For this review, take the finished solid that the model builds, in its own axes (mm). Face numbers are marked on the shaded views. A direction names the side the tool comes from. Round coordinates to 2 decimals unless told otherwise and drop trailing zeros. Loops run counter-clockwise (first coordinate to the right, second up) from the corner with the lowest first, then second, coordinate; pieces in that order, holes last.
1. Clearance check with flat-ended pins moving along their axes: pin 1 Ø13 at (x, z) = (35, 65) entering from +Y; pin 2 Ø1 at (x, z) = (-17.5, 28.5) entering from -Y; pin 3 Ø10 at (x, y) = (0, 0) entering from +Z; pin 4 Ø4 at (y, z) = (11, 114) entering from -X. State where each tip first meets the part, or that it passes through.
2. Consider section A-A on x = 0. State the section outline as (y, z) points.
3. Draft analysis for pull direction Y (two halves, no side actions). For the marked faces 4, 5 and 6, state which applies: released by +Y, released by -Y, zero draft, split by the parting line, or undercut.
4. Tool access review of the marked faces 1, 2 and 3: name each direction out of +Z, -Z, +X, -X, +Y, -Y from which nothing blocks a thin tool from reaching the whole face with its end or side.
5. Consider section C-C on y = 0. State the section outline as (x, z) points, then the cut area to 3 significant figures.
6. Consider section B-B on z = 65. State the section outline as (x, y) points.
7. To check wall thickness, follow line 1 along X through (y, z) = (46, 65); line 2 along Y through (x, z) = (-0.5, 136.5); line 3 along Z through (x, y) = (-2.5, 46). State the ranges of each line that lie inside material, in increasing order.
8. Consider section D-D on x = 35. State the section outline as (y, z) points.
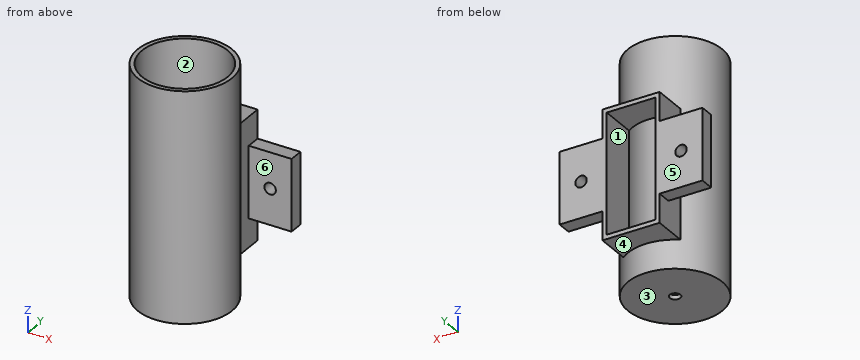
from build123d import *

# Parameters (mm, degrees)
SKETCH_1_R           = 33
EXTRUDE_1_DEPTH      = 160
SHELL_1_T            = -3
EXTRUDE_2_REACH      = 185.243
EXTRUDE_2_END_RADIUS = 33
SKETCH_2_W           = 40
SKETCH_2_H           = 90
SKETCH_3_W           = 34
SKETCH_3_H           = 84
CUT_EXTRUDE_1_DEPTH  = 60
SKETCH_4_W           = 50
SKETCH_4_H           = 10
EXTRUDE_3_DEPTH      = 30
SKETCH_5_R           = 4
CUT_EXTRUDE_2_DEPTH  = 30
SKETCH_6_W           = 50
SKETCH_6_H           = 10
EXTRUDE_4_DEPTH      = 30
SKETCH_7_R           = 4
CUT_EXTRUDE_3_DEPTH  = 30
SKETCH_8_R           = 3.75
CUT_EXTRUDE_4_DEPTH  = 10


with BuildPart() as part:
    # 草图1 → 凸台-拉伸1 (new body)
    with BuildSketch(Plane.XY):
        Circle(SKETCH_1_R)
    extrude(amount=EXTRUDE_1_DEPTH)

    # 抽壳1
    shell_1_openings = [part.faces().sort_by_distance(p)[0] for p in [
        (0, 0, 160),
    ]]
    offset(amount=SHELL_1_T, openings=shell_1_openings, kind=Kind.INTERSECTION)

    # 凸台-拉伸2: up to this cylinder (the profile starts outside it)
    extrude_2_end = Plane(origin=(0, 0, 65), z_dir=(0, 0, -1)) * Cylinder(EXTRUDE_2_END_RADIUS, 437.486, mode=Mode.PRIVATE)
    # 草图2 → 凸台-拉伸2 (add, up to the surface)
    with BuildSketch(Plane(origin=(0, 50, 0), x_dir=(1, 0, 0), z_dir=(0, 1, 0)), mode=Mode.PRIVATE) as extrude_2_sk1:
        with Locations((0, -65)):
            Rectangle(SKETCH_2_W, SKETCH_2_H)
    extrude_2_tool1 = extrude(extrude_2_sk1.sketch, amount=-EXTRUDE_2_REACH, mode=Mode.PRIVATE) - extrude_2_end
    add(extrude_2_tool1.solids().sort_by_distance((0, 50, 65))[0])

    # 草图3 → 切除-拉伸1 (cut)
    with BuildSketch(Plane(origin=(0, 50, 0), x_dir=(1, 0, 0), z_dir=(0, 1, 0))):
        with Locations((0, -65)):
            Rectangle(SKETCH_3_W, SKETCH_3_H)
    extrude(amount=-CUT_EXTRUDE_1_DEPTH, mode=Mode.SUBTRACT)

    # 草图4 → 凸台-拉伸3 (add)
    with BuildSketch(Plane.ZY.offset(20)):
        with Locations((65, 45)):
            Rectangle(SKETCH_4_W, SKETCH_4_H)
    extrude(amount=EXTRUDE_3_DEPTH)

    # 草图5 → 切除-拉伸2 (cut)
    with BuildSketch(Plane(origin=(0, 50, 0), x_dir=(1, 0, 0), z_dir=(0, 1, 0))):
        with Locations(Location((-35, -65, 0), (0, 0, 270))):
            Circle(SKETCH_5_R)
    extrude(amount=-CUT_EXTRUDE_2_DEPTH, mode=Mode.SUBTRACT)

    # 草图6 → 凸台-拉伸4 (add)
    with BuildSketch(Plane(origin=(20, 0, 0), x_dir=(0, 0, -1), z_dir=(1, 0, 0))):
        with Locations((-65, 45)):
            Rectangle(SKETCH_6_W, SKETCH_6_H)
    extrude(amount=EXTRUDE_4_DEPTH)

    # 草图7 → 切除-拉伸3 (cut)
    with BuildSketch(Plane(origin=(0, 50, 0), x_dir=(1, 0, 0), z_dir=(0, 1, 0))):
        with Locations(Location((35, -65, 0), (0, 0, 270))):
            Circle(SKETCH_7_R)
    extrude(amount=-CUT_EXTRUDE_3_DEPTH, mode=Mode.SUBTRACT)

    # 草图8 → 切除-拉伸4 (cut)
    with BuildSketch(Plane(origin=(0, 0, 0), x_dir=(-1, 0, 0), z_dir=(0, 0, -1))):
        Circle(SKETCH_8_R)
    extrude(amount=-CUT_EXTRUDE_4_DEPTH, mode=Mode.SUBTRACT)


solid = part.part
Resolved:
1. pin 1: stops at y = 50
1. pin 2: stops at y = -28.28
1. pin 3: stops at z = 3
1. pin 4: stops at x = -31.75
2. outline: (-33, 0) - (-3.75, 0) - (-3.75, 3) - (-30, 3) - (-30, 160) - (-33, 160) - close; (3.75, 0) - (33, 0) - (33, 20) - (50, 20) - (50, 23) - (30, 23) - (30, 3) - (3.75, 3) - close; (30, 107) - (50, 107) - (50, 110) - (33, 110) - (33, 160) - (30, 160) - close
3. face 4: zero draft
3. face 5: released by +Y
3. face 6: undercut
4. face 1: +Y
4. face 2: +Z
4. face 3: -Z, +X, -X, +Y, -Y
5. outline: (-33, 0) - (-3.75, 0) - (-3.75, 3) - (-30, 3) - (-30, 160) - (-33, 160) - close; (3.75, 0) - (33, 0) - (33, 160) - (30, 160) - (30, 3) - (3.75, 3) - close
5. area: 1,120 mm2
6. outline: (-50, 40) - (-39, 40) - (-39, 50) - (-50, 50) - close; (-31, 40) - (-20, 40) - (-20, 26.25) arc R33 ccw (long way) to (20, 26.25) - (20, 40) - (31, 40) - (31, 50) - (17, 50) - (17, 24.72) arc R30 cw (long way) to (-17, 24.72) - (-17, 50) - (-31, 50) - close; (39, 40) - (50, 40) - (50, 50) - (39, 50) - close
7. line 1: x = -50 to -39, -31 to -17, 17 to 31, 39 to 50
7. line 2: y = -33 to -30, 30 to 33
7. line 3: z = 20 to 23, 107 to 110
8. outline: (40, 40) - (50, 40) - (50, 61) - (40, 61) - close; (40, 69) - (50, 69) - (50, 90) - (40, 90) - close
